For this review, use the dimensioned drawing (mm, ordinates from the lowest corner) and the shaded views. A direction names the side the tool comes from. Give positions to 0.01 mm unless a question says otherwise; leave off trailing zeros. Loops run counter-clockwise (first coordinate to the right, second up) from the corner with the lowest first, then second, coordinate; pieces in that order, holes last. Notation, with made-up numbers: M 28,54 L 34,54 A20 cw 34,87 Z; hole C -12,73 d3. An arc over 180 degrees is marked long. Use a Markdown table: item, result. Add a question column.
(1) For the marked faces 1 and 2, list the 3-axis set-ups (+Z, -Z, +X, -X, +Y, -Y) from which the entire face can be reached by the end or side of a thin tool; tool diameter is ignored.
(2) Insertion check: pin 1 Ø3.5 at (x, y) = (5, 18) entering from +Z; pin 2 Ø1.8 at (x, y) = (25, 18) entering from +Z; pin 3 Ø6 at (x, z) = (20.5, 17.5) entering from +Y; pin 4 Ø3 at (x, z) = (21, 11.5) entering from -Y. Each pin has a flat end and moves straight along its axis. Give the tip position at first contact, or say it passes through.
(3) Add section A-A, the plane y = 18. Give the boundary of the cut face in (x, z).
(4) Add section B-B, the plane x = 5. Give the boundary of the cut face in (y, z), then the cut area to 3 significant figures.
(5) Add section D-D, the plane z = 10.75. Give the boundary of the cut face in (x, y).
(6) Draft analysis for pull direction Z (two halves, no side actions). For the marked faces 3, 4 and 5, state which applies: pulls with the +Z half, pulls with the -Z half, needs draft (parallel to the pull), parting line crosses it, or undercut.
(7) For probe 1 along X at (y, z) = (2.1, 18); probe 2 along Y at (x, z) = (25, 0.9); probe 3 along Y at (x, z) = (1.5, 10.5), list the stretches that pass through material, from the lowest coordinate up.
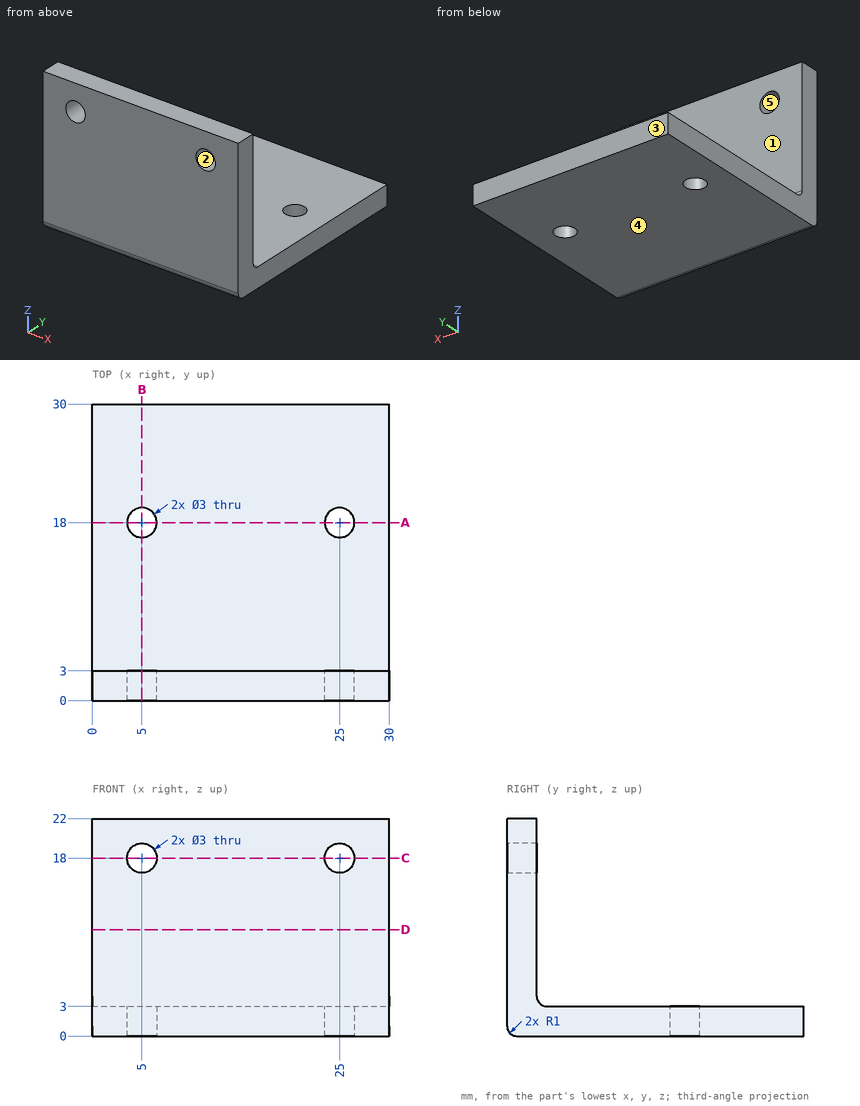
Established:
| question | item | result |
|---|---|---|
| 1 | face 1 | +Z, +X, -X, +Y |
| 1 | face 2 | +Y, -Y |
| 2 | pin 1 | z = 3 |
| 2 | pin 2 | through |
| 2 | pin 3 | y = 3 |
| 2 | pin 4 | y = 0 |
| 3 | outline | M 0,0 L 3.5,0 L 3.5,3 L 0,3 Z; M 6.5,0 L 23.5,0 L 23.5,3 L 6.5,3 Z; M 26.5,0 L 30,0 L 30,3 L 26.5,3 Z |
| 4 | outline | M 0,1 A1 ccw 1,0 L 16.5,0 L 16.5,3 L 4,3 A1 cw 3,4 L 3,16.5 L 0,16.5 Z; M 0,19.5 L 3,19.5 L 3,22 L 0,22 Z; M 19.5,0 L 30,0 L 30,3 L 19.5,3 Z |
| 4 | area | 129 mm^2 |
| 5 | outline | M 0,0 L 30,0 L 30,3 L 0,3 Z |
| 6 | face 3 | needs draft |
| 6 | face 4 | pulls with the -Z half |
| 6 | face 5 | undercut |
| 7 | probe 1 | 0 to 3.5, 6.5 to 23.5, 26.5 to 30 |
| 7 | probe 2 | 0.01 to 16.5, 19.5 to 30 |
| 7 | probe 3 | 0 to 3 |
